Here's the drawing with two shaded views (mm, measured from the low corner). I have some questions. A direction names the side the tool comes from. Give positions to 0.01 mm unless a question says otherwise; leave off trailing zeros. Write each loop counter-clockwise with the first axis right and the second up, starting at its lowest first coordinate (ties: lowest second). Pieces come first, ordered by that corner, then holes. Notation, with made-up numbers: M 57,20.25 L 84,20.25 A23 cw 84,59.25 Z; hole C 26,69.25 d4. An arc over 180 degrees is marked long. Use one line per item in the form item = value. Start each with the question number.
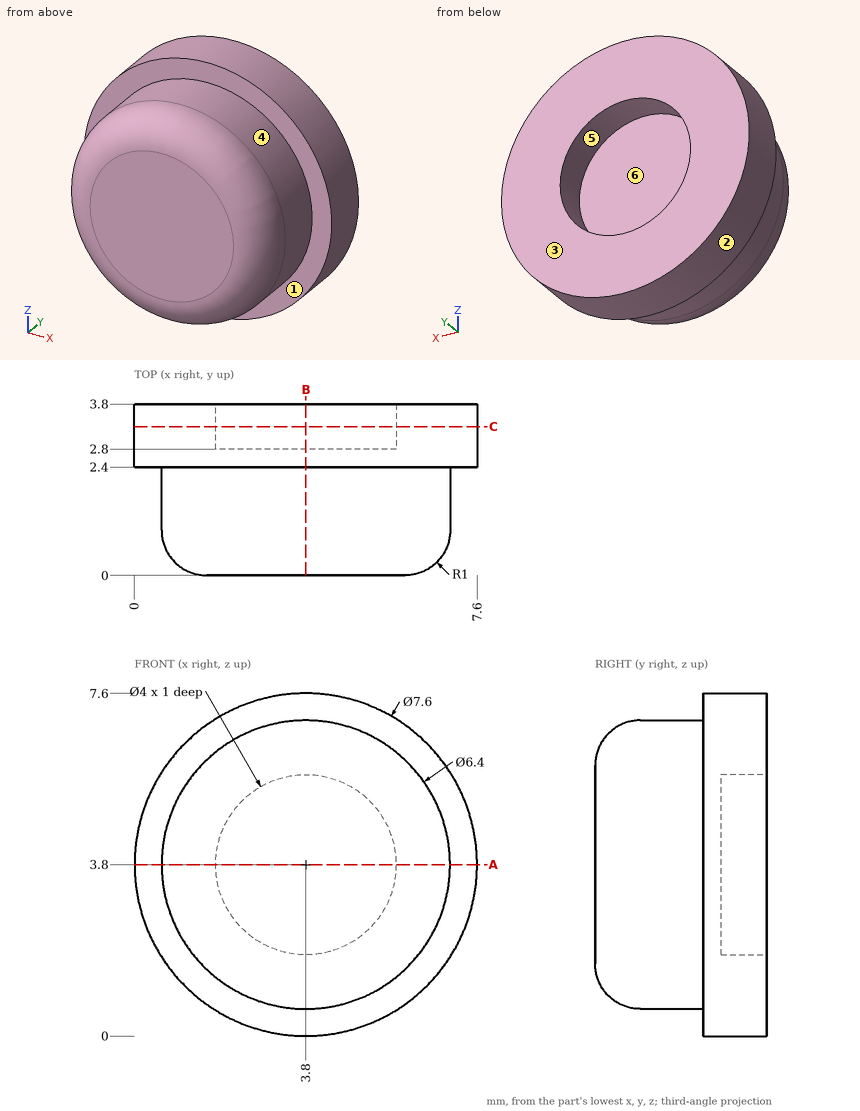
1) Suppose I cut it at B-B, the plane x = 3.8. List the corners of the cut face in (y, z) for me.
2) On a 3-axis mill with a long thin cutter (end or side, diameter ignored), from which of +Z, -Z, +X, -X, +Y, -Y can I reach the whole of each face in a straight line? I mean the marked faces 1 and 2. Say none if no direction works.
3) Will this pin go through, and if not, where does the flat tip stop? P1, Ø1, axis at y = 1, z = 3, coming from the +X side.
4) Suppose I cut it at A-A, the plane z = 3.8. List the corners of the cut face in (x, y) for me, and give its area (3 significant figures).
5) Thinking about a two-plate mould opening in Z: for the marked faces 3, 4, 5 and 6, which applies, released by +Z, released by -Z, zero draft, split by the parting line, or undercut?
6) Please list where these lines run through material, in increasing order: line 1 (Z direction, x = 5.5, y = 3.3); line 2 (Y direction, x = 4.5, z = 5.5); line 3 (X direction, y = 3.6, z = 2.25).
7) Suppose I cut it at C-C, the plane y = 3.3. List the corners of the cut face in (x, z) for me.
Checks:
q1.outline = M 0,1.6 A1 ccw 1,0.6 L 2.4,0.6 L 2.4,0 L 3.8,0 L 3.8,1.8 L 2.8,1.8 L 2.8,5.8 L 3.8,5.8 L 3.8,7.6 L 2.4,7.6 L 2.4,7 L 1,7 A1 ccw 0,6 Z
q2.face_1 = -Y
q2.face_2 = +Y, -Y
q3.P1 = 6.99
q4.outline = M 0,2.4 L 0.6,2.4 L 0.6,1 A1 ccw 1.6,0 L 6,0 A1 ccw 7,1 L 7,2.4 L 7.6,2.4 L 7.6,3.8 L 5.8,3.8 L 5.8,2.8 L 1.8,2.8 L 1.8,3.8 L 0,3.8 Z
q4.area = 21.6 mm^2
q5.face_3 = zero draft
q5.face_4 = split by the parting line
q5.face_5 = undercut
q5.face_6 = undercut
q6.line_1 = 0.4 to 2.75, 4.85 to 7.2
q6.line_2 = 0 to 2.8
q6.line_3 = 0.33 to 2.54, 5.06 to 7.27
q7.outline = C 3.8,3.8 d7.6; hole C 3.8,3.8 d4
